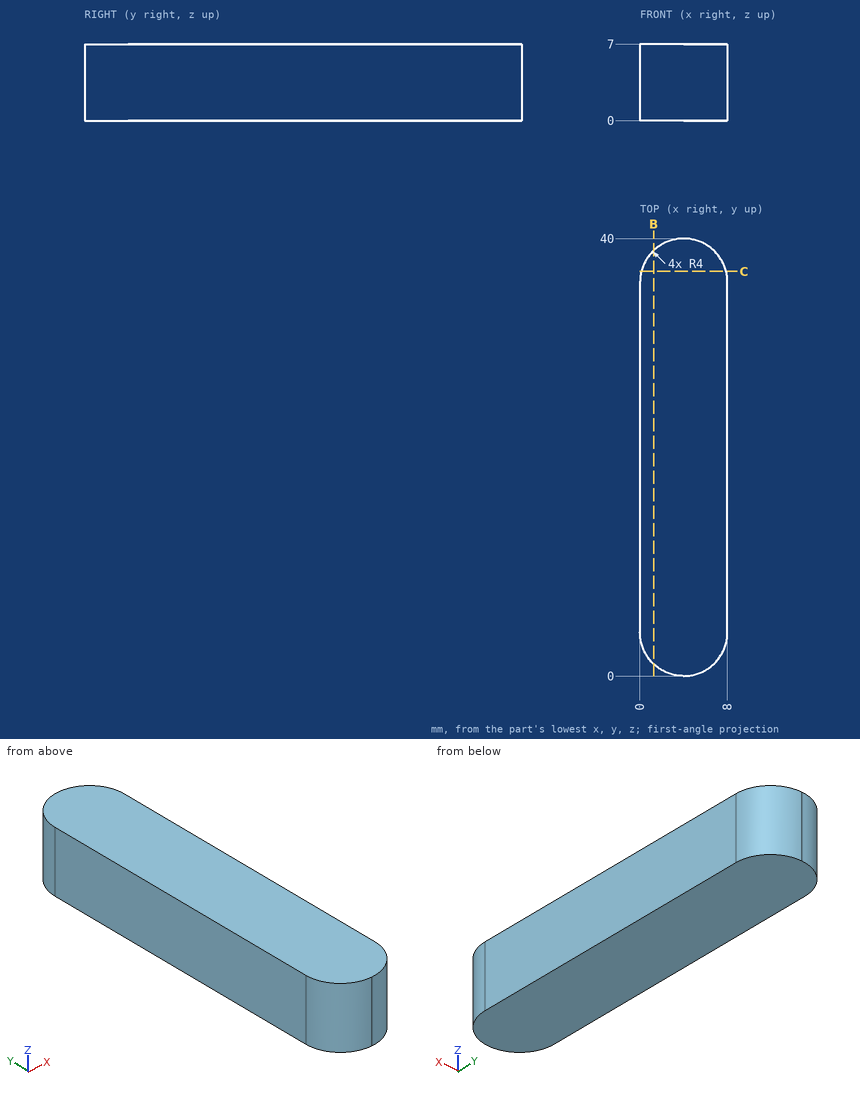
Design review of the part shown in the three views and the two pictorial views. Dimensions are in mm from the part's minimum x, y and z. Round coordinates to 2 decimals unless told otherwise and drop trailing zeros. Loops run counter-clockwise (first coordinate to the right, second up) from the corner with the lowest first, then second, coordinate; pieces in that order, holes last. Notation, with made-up numbers: (9.25, 0) - (47.25, 0) arc R15 cw to (47.25, 4) - close; hole circle Ø9 at (-33, 26.5). An arc over 180 degrees is marked (long way). Answer as CSV lines item,"result".
(1) Wall thickness on line 1 (Y direction, x = 3.75, z = 5.5); line 2 (Y direction, x = 6.5, z = 2.5); line 3 (X direction, y = 38, z = 0.5) (1 decimal): over which ranges is each line inside the solid? List them lowest first.
Checked values:
line 1,"y = 0.01 to 39.99"
line 2,"y = 0.88 to 39.12"
line 3,"x = 0.5 to 7.5"
(2) Consider section C-C on y = 37. Give the boundary of the cut face in (x, z).
Checked values:
outline,"(0.13, 0) - (7.87, 0) - (7.87, 7) - (0.13, 7) - close"
(3) Consider section B-B on x = 1.25. Give the boundary of the cut face in (y, z) (1 decimal), then the cut area to 3 significant figures.
Checked values:
outline,"(1.1, 0) - (38.9, 0) - (38.9, 7) - (1.1, 7) - close"
area,"265 mm2"
